```python
from build123d import *

# Parameters (mm, degrees)
SKETCH1_R           = 15.5
SKETCH1_R_2         = 14.5
BOSS_EXTRUDE1_DEPTH = 117


with BuildPart() as part:
    # Sketch1 → Boss-Extrude1 (new body)
    with BuildSketch(Plane.XY):
        Circle(SKETCH1_R)
        Circle(SKETCH1_R_2, mode=Mode.SUBTRACT)
    extrude(amount=BOSS_EXTRUDE1_DEPTH)

    # Sketch4 → Revolve1 (revolve)
    with BuildSketch(Plane(origin=(0, 0, 0), x_dir=(0, 0, -1), z_dir=(1, 0, 0)), mode=Mode.PRIVATE) as revolve1_sk:
        Polygon((0, -15.5), (4.3, -4.75), (11.8, -4.75), (11.8, 0), (4.3, 0), (3.3, 0), (3.3, -4.75), (0, -13), align=None)
    revolve(revolve1_sk.sketch.rotate(Axis((0, 0, 0), (0, 0, -1)), 270), axis=Axis((0, 0, 0), (0, 0, -1)))


solid = part.part
```
Source: CAD feature listing. Evaluate the final solid. Frame: model axes, mm. A direction names the side the tool comes from. Coordinates: 2 decimals unless noted, no trailing zeros. Order: outer loops, then holes, each group sorted by start corner. A loop starts at its lowest first (then second) coordinate and runs counter-clockwise, first axis right, second up. Notation, with made-up numbers: M -26.75,75.25 L -13.75,75.25 A32 ccw -13.75,110.25 Z; hole C 6.5,-10 d11. An arc over 180 degrees is marked long. Write each question's results on one line, items separated by ' | '. Start each with the question number.
1) Line query: line 1 (Y direction, x = 0, z = 59.5); line 2 (X direction, y = -3.5, z = 111); line 3 (X direction, y = 7.5, z = 9.5). Output: solid intervals per line, ascending. Write a range as from..to.
2) Section query A-A (z = 3). Return the cut outline in (x, y), plus the area to 3 significant figures.
3) Section query B-B (y = 0). Return the cut outline in (x, z), plus the area to 3 significant figures.
4) Access query for faces 4 (the face through (-2.018, 15.368, 57.681)), 5 (the face through (0, 0, -3.3)). Directions: +Z, -Z, +X, -X, +Y, -Y. A direction counts if a zero-diameter tool reaches every point of the face in a straight line with its end or side. Return the directions, or none.
5) Draft query along Y for faces 1 (the face through (9, -10, 0)), 2 (the face through (6, -14, 117)), 3 (the face through (-3.77, 2.89, -8.1)). Return one class per face: released by +Y, released by -Y, zero draft, split by the parting line, or undercut.
6) Contact query for flat-ended pins moving along their axis: pin 1 Ø10 at (x, y) = (7.5, 10) entering from -Z; pin 2 Ø1 at (y, z) = (3.5, 64.5) entering from -X; pin 3 Ø4 at (x, y) = (3.5, 7) entering from -Z. Output: stop coordinate, or through.
Answers:
1) line 1: y = -15.5..-14.5, 14.5..15.5 | line 2: x = -15.1..-14.07, 14.07..15.1 | line 3: x = -13.56..-12.41, 12.41..13.56
2) outline: C 0,0 d31; hole C 0,0 d29 | area: 94.2 mm^2
3) outline: M -15.5,0 L -4.75,-4.3 L -4.75,-11.8 L 4.75,-11.8 L 4.75,-4.3 L 15.5,0 L 15.5,117 L 14.5,117 L 14.5,0 L 13,0 L 4.75,-3.3 L -4.75,-3.3 L -13,0 L -14.5,0 L -14.5,117 L -15.5,117 Z | area: 334 mm^2
4) face 4: +Z, -Z | face 5: +Z
5) face 1: undercut | face 2: zero draft | face 3: split by the parting line
6) pin 1: stops at z = -3.2 | pin 2: stops at x = -15.21 | pin 3: stops at z = -3.87
